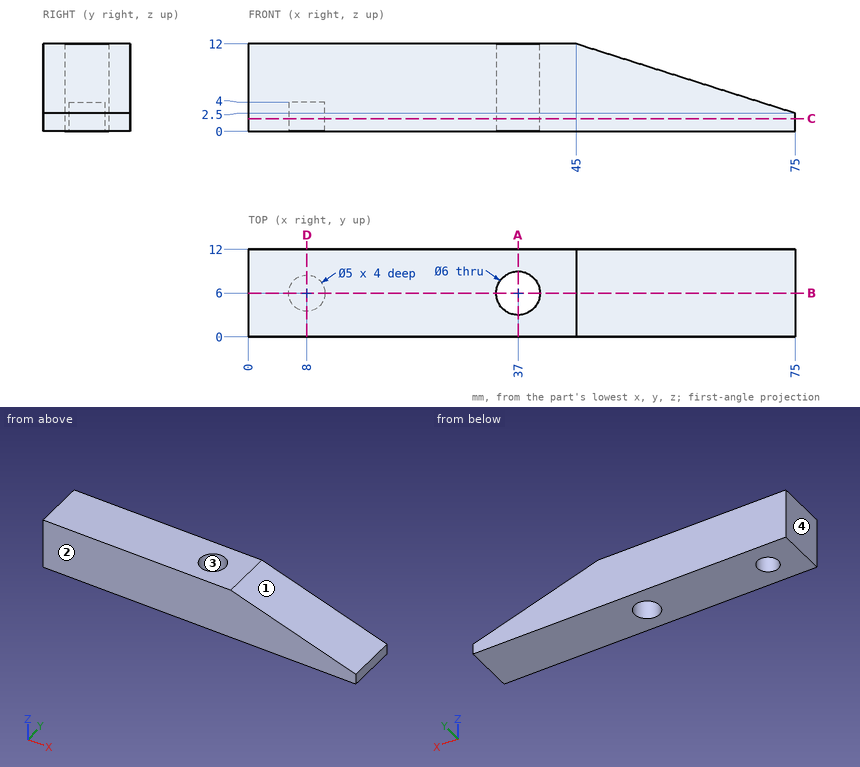
Input: dimensioned drawing with shaded views. Units: mm. Origin: part minimum x, y, z. Coordinates: 2 decimals unless noted, no trailing zeros. Order: outer loops, then holes, each group sorted by start corner. A loop starts at its lowest first (then second) coordinate and runs counter-clockwise, first axis right, second up. Notation, with made-up numbers: (32, -29) - (88, -29) arc R31 ccw to (88, 8) - close; hole circle Ø1 at (72, -1.75). An arc over 180 degrees is marked (long way). Return JSON: item names as keys, results as strings. Group by question number.
1. Material intervals for line 1 along X through (y, z) = (6, 2.05); line 2 along Y through (x, z) = (37, 4.5); line 3 along Y through (x, z) = (8, 2.9), sorted ascending. Write a range as [from, to].
2. Cut plane C-C (z = 1.75). Output: boundary loops of the cut face in (x, y), plus the area to 3 significant figures.
3. Cut plane B-B (y = 6). Output: boundary loops of the cut face in (x, z).
4. Pin query (flat end, axial travel): pin 1 (3.5 mm diameter, centred on x = 37, y = 6, fed in from +Z). Return the tip coordinate at first contact, or that it passes through.
5. Cut plane D-D (x = 8). Output: boundary loops of the cut face in (y, z), plus the area to 3 significant figures.
6. Pull-direction query (X, two-part tool) for the marked faces 1, 2, 3 and 4; classes: pulls with the +X half, pulls with the -X half, needs draft (parallel to the pull), parting line crosses it, or undercut.
7. Cut plane A-A (x = 37). Output: boundary loops of the cut face in (y, z).
Resolved:
{
 "1": {"line 1": "x = [0, 5.5], [10.5, 34], [40, 75]", "line 2": "y = [0, 3], [9, 12]", "line 3": "y = [0, 3.5], [8.5, 12]"},
 "2": {"outline": "(0, 0) - (75, 0) - (75, 12) - (0, 12) - close; hole circle Ø5 at (8, 6); hole circle Ø6 at (37, 6)", "area": "852 mm²"},
 "3": {"outline": "(0, 0) - (5.5, 0) - (5.5, 4) - (10.5, 4) - (10.5, 0) - (34, 0) - (34, 12) - (0, 12) - close; (40, 0) - (75, 0) - (75, 2.5) - (45, 12) - (40, 12) - close"},
 "4": {"pin 1": "passes through"},
 "5": {"outline": "(0, 0) - (3.5, 0) - (3.5, 4) - (8.5, 4) - (8.5, 0) - (12, 0) - (12, 12) - (0, 12) - close", "area": "124 mm²"},
 "6": {"face 1": "pulls with the +X half", "face 2": "needs draft", "face 3": "undercut", "face 4": "pulls with the -X half"},
 "7": {"outline": "(0, 0) - (3, 0) - (3, 12) - (0, 12) - close; (9, 0) - (12, 0) - (12, 12) - (9, 12) - close"}
}
